```python
from build123d import *

# Parameters (mm, degrees)
BOSS_EXTRUDE1_DEPTH = 14.1


with BuildPart() as part:
    # Esboço1 → Boss-Extrude1 (new body)
    with BuildSketch(Plane.XY):
        with BuildLine():
            Line((0, 0), (14.098810584, 0))
            Line((14.098810584, 0), (14.098810584, -6))
            ThreePointArc((14.098810584, -6), (13.648810584, -6.45), (13.198810584, -6))
            Line((13.198810584, -6), (13.198810584, -1.6))
            Line((13.198810584, -1.6), (11.898810584, -1.6))
            Line((11.898810584, -1.6), (11.898810584, -6))
            ThreePointArc((11.898810584, -6), (11.448810584, -6.45), (10.998810584, -6))
            Line((10.998810584, -6), (10.998810584, -1.6))
            Line((10.998810584, -1.6), (9.698810584, -1.6))
            Line((9.698810584, -1.6), (9.698810584, -6))
            ThreePointArc((9.698810584, -6), (9.249405292, -6.449405292), (8.8, -6))
            Line((8.8, -6), (8.8, -1.6))
            Line((8.8, -1.6), (7.5, -1.6))
            Line((7.5, -1.6), (7.5, -6))
            ThreePointArc((7.5, -6), (7.05, -6.45), (6.6, -6))
            Line((6.6, -6), (6.6, -1.6))
            Line((6.6, -1.6), (5.3, -1.6))
            Line((5.3, -1.6), (5.3, -6))
            ThreePointArc((5.3, -6), (4.85, -6.45), (4.4, -6))
            Line((4.4, -6), (4.4, -1.6))
            Line((4.4, -1.6), (3.1, -1.6))
            Line((3.1, -1.6), (3.1, -6))
            ThreePointArc((3.1, -6), (2.65, -6.45), (2.2, -6))
            Line((2.2, -6), (2.2, -1.6))
            Line((2.2, -1.6), (0.9, -1.6))
            Line((0.9, -1.6), (0.9, -6))
            ThreePointArc((0.9, -6), (0.45, -6.45), (0, -6))
            Line((0, -6), (0, 0))
        make_face()
    extrude(amount=BOSS_EXTRUDE1_DEPTH)


solid = part.part
```
Input: part model. Units: mm. Frame: model coordinates. A direction names the side the tool comes from. Round coordinates to 2 decimals unless told otherwise and drop trailing zeros. Loops run counter-clockwise (first coordinate to the right, second up) from the corner with the lowest first, then second, coordinate; pieces in that order, holes last. Notation, with made-up numbers: (71.25, 9) -> (114.25, 9) arc R22 ccw to (114.25, 42) -> close; hole circle Ø4 at (32.5, -12.5). An arc over 180 degrees is marked (long way). Write each question's results on one line, items separated by ' | '.
1. Ray query, line 1 (Y direction, x = 3.5, z = 11.25); line 2 (Y direction, x = 11.5, z = 10.5). Return the intervals inside material, ascending. Write a range as from..to.
Geometry results:
line 1: -1.6..0 | line 2: -6.45..0
2. Section A-A (y = -4.25). Return loops of the section in (x, z), and give its area (3 significant figures).
Geometry results:
outline: (0, 0) -> (0.9, 0) -> (0.9, 14.1) -> (0, 14.1) -> close; (2.2, 0) -> (3.1, 0) -> (3.1, 14.1) -> (2.2, 14.1) -> close; (4.4, 0) -> (5.3, 0) -> (5.3, 14.1) -> (4.4, 14.1) -> close; (6.6, 0) -> (7.5, 0) -> (7.5, 14.1) -> (6.6, 14.1) -> close; (8.8, 0) -> (9.7, 0) -> (9.7, 14.1) -> (8.8, 14.1) -> close; (11, 0) -> (11.9, 0) -> (11.9, 14.1) -> (11, 14.1) -> close; (13.2, 0) -> (14.1, 0) -> (14.1, 14.1) -> (13.2, 14.1) -> close | area: 88.8 mm2
3. Set-up query: faces 4 (the face through (0.9, -4, 7)), 5 (the face through (0, -3, 7)). Return all of +Z, -Z, +X, -X, +Y, -Y with unobstructed straight access to the full face (end or side cutting, diameter ignored); none if empty.
Geometry results:
face 4: +Z, -Z, -Y | face 5: +Z, -Z, -X, +Y, -Y
4. First-contact query: P1, Ø1, axis at x = 10, z = 9.5, coming from the -Y side. Flat tip, straight axial feed; report the tip coordinate or a pass-through.
Geometry results:
P1: y = -6.37
5. Section B-B (z = 8.75). Return loops of the section in (x, y).
Geometry results:
outline: (0, -6) arc R0.45 ccw to (0.9, -6) -> (0.9, -1.6) -> (2.2, -1.6) -> (2.2, -6) arc R0.45 ccw to (3.1, -6) -> (3.1, -1.6) -> (4.4, -1.6) -> (4.4, -6) arc R0.45 ccw to (5.3, -6) -> (5.3, -1.6) -> (6.6, -1.6) -> (6.6, -6) arc R0.45 ccw to (7.5, -6) -> (7.5, -1.6) -> (8.8, -1.6) -> (8.8, -6) arc R0.45 ccw to (9.7, -6) -> (9.7, -1.6) -> (11, -1.6) -> (11, -6) arc R0.45 ccw to (11.9, -6) -> (11.9, -1.6) -> (13.2, -1.6) -> (13.2, -6) arc R0.45 ccw to (14.1, -6) -> (14.1, 0) -> (0, 0) -> close
6. Mould query, pull axis X, two halves, no side actions, for faces 1 (the face through (9.699, -4, 7)), 2 (the face through (7, 0, 7)), 3 (the face through (14.099, -3, 7)). Classes: +X half, -X half, draft (parallel to the pull), parting line (faces both ways), or undercut.
Geometry results:
face 1: undercut | face 2: draft | face 3: +X half
